Part model, mm, in its own coordinate system. A direction names the side the tool comes from. Coordinates: 2 decimals unless noted, no trailing zeros. Loops run counter-clockwise (first coordinate to the right, second up) from the corner with the lowest first, then second, coordinate; pieces in that order, holes last. Notation, with made-up numbers: (72.25, 49.5) -> (78.25, 49.5) arc R19 ccw to (78.25, 69.5) -> close; hole circle Ø9 at (29.5, -23.5). An arc over 180 degrees is marked (long way). One line per question, with ' | ' between items. Start each with the question number.
1) Probe L1, parallel to Y at x = 0, z = 1.1; L2, parallel to Y at x = 18.5, z = 3.85; L3, parallel to X at y = 15.5, z = 0.55. List the from-to ranges inside material, lowest first. Write a range as from..to.
2) Drop flat-ended pins along their axis: pin 1 (1.6 mm diameter, centred on x = 0, y = 15.35, fed in from +Z); pin 2 (20 mm diameter, centred on x = 1.5, y = 1, fed in from +Z); pin 3 (2.5 mm diameter, centred on x = -17, y = 15.35, fed in from +Z); pin 4 (1.2 mm diameter, centred on x = -7.5, z = 2, fed in from -Y). Give the stop position or say it passes through.
3) Cut at B-B (y = 0.35). List the corners of the cut face in (x, z).
4) Cut at A-A (z = 2). List the corners of the cut face in (x, y), plus the area to 3 significant figures.
5) Two-plate mould, pull along X, no slides. Class faces 1 (the face through (0.54, 16.19, 1.97)), 2 (the face through (-20, -0.2, 0.6)), 3 (the face through (0, 0, 0)): released by +X, released by -X, zero draft, split by the parting line, or undercut.
6) 3-axis set-ups, long thin cutter, end or side, ignore diameter. For faces 4 (the face through (-0.3, 16.5, 4)), 5 (the face through (0, 1, 1)), 6 (the face through (7, -14.85, 2)): which of +Z, -Z, +X, -X, +Y, -Y reach the whole face in a straight line?
7) Cut at D-D (y = 15.35). List the corners of the cut face in (x, z), plus the area to 3 significant figures.
8) Cut at C-C (x = 12.5). List the corners of the cut face in (y, z), plus the area to 3 significant figures.
from build123d import *

# Parameters (mm, degrees)
SKETCH1_W           = 40
SKETCH1_H           = 35.7
SKETCH1_R           = 1
BOSS_EXTRUDE1_DEPTH = 4
SKETCH2_W           = 50
SKETCH2_H           = 25
CUT_EXTRUDE1_DEPTH  = 3
SKETCH3_R           = 1
CUT_EXTRUDE2_DEPTH  = 3
SKETCH4_R           = 5
CUT_EXTRUDE3_DEPTH  = 28.103920381


with BuildPart() as part:
    # Sketch1 → Boss-Extrude1 (new body)
    with BuildSketch(Plane.XY):
        Rectangle(SKETCH1_W, SKETCH1_H)
        with Locations((-17, 15.35)):
            Circle(SKETCH1_R, mode=Mode.SUBTRACT)
        with Locations((0, 15.35)):
            Circle(SKETCH1_R, mode=Mode.SUBTRACT)
        with Locations((17, 15.35)):
            Circle(SKETCH1_R, mode=Mode.SUBTRACT)
        with Locations((-17, -14.65)):
            Circle(SKETCH1_R, mode=Mode.SUBTRACT)
        with Locations((0, -14.65)):
            Circle(SKETCH1_R, mode=Mode.SUBTRACT)
        with Locations((17, -14.65)):
            Circle(SKETCH1_R, mode=Mode.SUBTRACT)
    extrude(amount=BOSS_EXTRUDE1_DEPTH)

    # Sketch2 → Cut-Extrude1 (cut)
    with BuildSketch(Plane.XY.offset(4)):
        with Locations((0, 0.35)):
            Rectangle(SKETCH2_W, SKETCH2_H)
    extrude(amount=-CUT_EXTRUDE1_DEPTH, mode=Mode.SUBTRACT)

    # Sketch3 → Cut-Extrude2 (cut)
    with BuildSketch(Plane.XZ.offset(17.85)):
        with Locations((-7.5, 2)):
            Circle(SKETCH3_R)
        with Locations((7.5, 2)):
            Circle(SKETCH3_R)
    extrude(amount=-CUT_EXTRUDE2_DEPTH, mode=Mode.SUBTRACT)

    # Sketch4 → Cut-Extrude3 (cut, through all)
    with BuildSketch(Plane(origin=(0, 0, 0), x_dir=(-1, 0, 0), z_dir=(0, 0, -1))):
        with Locations((-12.5, 0.35)):
            Circle(SKETCH4_R)
    extrude(amount=-CUT_EXTRUDE3_DEPTH, mode=Mode.SUBTRACT)


solid = part.part
Reported:
1) L1: y = -17.85..-15.65, -13.65..-12.15, 12.85..14.35, 16.35..17.85 | L2: y = -17.85..-12.15, 12.85..17.85 | L3: x = -20..-17.99, -16.01..-0.99, 0.99..16.01, 17.99..20
2) pin 1: passes through | pin 2: stops at z = 1 | pin 3: stops at z = 4 | pin 4: stops at y = -14.85
3) outline: (-20, 0) -> (7.5, 0) -> (7.5, 1) -> (-20, 1) -> close; (17.5, 0) -> (20, 0) -> (20, 1) -> (17.5, 1) -> close
4) outline: (-20, -17.85) -> (-8.5, -17.85) -> (-8.5, -14.85) -> (-6.5, -14.85) -> (-6.5, -17.85) -> (6.5, -17.85) -> (6.5, -14.85) -> (8.5, -14.85) -> (8.5, -17.85) -> (20, -17.85) -> (20, -12.15) -> (-20, -12.15) -> close; (-20, 12.85) -> (20, 12.85) -> (20, 17.85) -> (-20, 17.85) -> close; hole circle Ø2 at (-17, -14.65); hole circle Ø2 at (-17, 15.35); hole circle Ø2 at (0, -14.65); hole circle Ø2 at (0, 15.35); hole circle Ø2 at (17, -14.65); hole circle Ø2 at (17, 15.35) | area: 397 mm²
5) face 1: undercut | face 2: released by -X | face 3: zero draft
6) face 4: +Z, +X, -X, +Y, -Y | face 5: +Z, +X, -X | face 6: -Y
7) outline: (-20, 0) -> (-18, 0) -> (-18, 4) -> (-20, 4) -> close; (-16, 0) -> (-1, 0) -> (-1, 4) -> (-16, 4) -> close; (1, 0) -> (16, 0) -> (16, 4) -> (1, 4) -> close; (18, 0) -> (20, 0) -> (20, 4) -> (18, 4) -> close | area: 136 mm²
8) outline: (-17.85, 0) -> (-4.65, 0) -> (-4.65, 1) -> (-12.15, 1) -> (-12.15, 4) -> (-17.85, 4) -> close; (5.35, 0) -> (17.85, 0) -> (17.85, 4) -> (12.85, 4) -> (12.85, 1) -> (5.35, 1) -> close | area: 57.8 mm²
